```python
from build123d import *

# Parameters (mm, degrees)
F1_DEPTH = 3.048


with BuildPart() as f1:
    # F0 (on Front) → F1 (new body)
    with BuildSketch(Plane.XZ):
        with BuildLine():
            add(Edge.make_bspline(
                [(0, -29.2028061362), (0.1994290432, -29.2090684708), (0.3988582249, -29.2153378493), (0.5982729839, -29.2216137104)],
                knots=[0, 0, 0, 0, 0.0080246695, 0.0080246695, 0.0080246695, 0.0080246695], degree=3))
            Line((0, -29.2028061362), (0, -38.7278061362))
            Line((0, -38.7278061362), (9.525, -38.7278061362))
            ThreePointArc((9.525, -38.7278061362), (6.9434924632, -32.2075655415), (0.5982729839, -29.2216137104))
        make_face()
        with BuildLine():
            ThreePointArc((-9.525, -38.7278061362), (-6.7351920908, -31.9926140454), (0, -29.2028061362))
            Line((0, -29.2028061362), (0, -15.875))
            ThreePointArc((0, -15.875), (-11.0057082375, -11.4407172498), (-15.8630798211, -0.6150801499))
            add(Edge.make_bspline(
                [(-15.8630798211, -0.6150801499), (-15.5610688303, -14.0326352056), (-12.5430344151, -26.3802206709), (-9.525, -38.7278061362)],
                knots=[0.5347471817, 0.5347471817, 0.5347471817, 0.5347471817, 1, 1, 1, 1], degree=3))
        make_face()
        with BuildLine():
            Line((0, -38.7278061362), (0, -29.2028061362))
            ThreePointArc((0, -29.2028061362), (-6.7351920908, -31.9926140454), (-9.525, -38.7278061362))
            ThreePointArc((-9.525, -38.7278061362), (-6.7351920908, -45.4629982271), (0, -48.2528061362))
            add(Edge.make_bspline(
                [(0, -48.2528061362), (0.2131130588, -48.2456482665), (0.4262259719, -48.2384878681), (0.6393387432, -48.2313250094)],
                knots=[0, 0, 0, 0, 0.6396952306, 0.6396952306, 0.6396952306, 0.6396952306], degree=3))
            ThreePointArc((0.6393387432, -48.2313250094), (6.957561589, -45.2330318614), (9.525, -38.7278061362))
            Line((9.525, -38.7278061362), (0, -38.7278061362))
        make_face()
        with BuildLine():
            Line((0, -15.875), (0, -29.2028061362))
            ThreePointArc((0, -29.2028061362), (0.2992842663, -29.2075091909), (0.5982729839, -29.2216137104))
            add(Edge.make_bspline(
                [(0.5982729839, -29.2216137104), (4.3416181778, -29.339422014), (8.0798811955, -29.4595146085), (11.716745228, -29.5781777813)],
                knots=[0.0080246695, 0.0080246695, 0.0080246695, 0.0080246695, 0.1586610028, 0.1586610028, 0.1586610028, 0.1586610028], degree=3))
            add(Edge.make_bspline(
                [(15.8630798211, -0.6150801499), (15.6355353264, -10.7242843795), (13.866216965, -20.2261112434), (11.7167452282, -29.578177782)],
                knots=[0.5347471817, 0.5347471817, 0.5347471817, 0.5347471817, 0.8852831578, 0.8852831578, 0.8852831578, 0.8852831578], degree=3))
            ThreePointArc((15.8630798211, -0.6150801499), (11.0057082375, -11.4407172498), (0, -15.875))
        make_face()
        with BuildLine():
            ThreePointArc((0.5982729839, -29.2216137104), (0.2992842663, -29.2075091909), (0, -29.2028061362))
            add(Edge.make_bspline(
                [(0, -29.2028061362), (0.1994290432, -29.2090684708), (0.3988582249, -29.2153378493), (0.5982729839, -29.2216137104)],
                knots=[0, 0, 0, 0, 0.0080246695, 0.0080246695, 0.0080246695, 0.0080246695], degree=3))
        make_face()
        with BuildLine():
            ThreePointArc((-15.8630798211, -0.6150801499), (-11.0057082375, -11.4407172498), (0, -15.875))
            Line((0, -15.875), (0, 0))
            Line((0, 0), (0, 15.875))
            ThreePointArc((0, 15.875), (-11.2253201513, 11.2253201513), (-15.875, 0))
            add(Edge.make_bspline(
                [(-15.875, 0), (-15.8716656679, -0.2052784728), (-15.8676890566, -0.4103039216), (-15.8630798211, -0.6150801499)],
                knots=[0.5276465798, 0.5276465798, 0.5276465798, 0.5276465798, 0.5347471817, 0.5347471817, 0.5347471817, 0.5347471817], degree=3))
        make_face()
        with BuildLine():
            Line((0, 0), (0, -15.875))
            ThreePointArc((0, -15.875), (11.0057082375, -11.4407172498), (15.8630798211, -0.6150801499))
            add(Edge.make_bspline(
                [(15.875, 0), (15.8716656679, -0.2052784728), (15.8676890566, -0.4103039216), (15.8630798211, -0.6150801499)],
                knots=[0.5276465798, 0.5276465798, 0.5276465798, 0.5276465798, 0.5347471817, 0.5347471817, 0.5347471817, 0.5347471817], degree=3))
            ThreePointArc((15.875, 0), (11.2253201513, 11.2253201513), (0, 15.875))
            Line((0, 15.875), (0, 0))
        make_face()
        with BuildLine():
            add(Edge.make_bspline(
                [(0.5982729839, -29.2216137104), (4.3416181778, -29.339422014), (8.0798811955, -29.4595146085), (11.716745228, -29.5781777813)],
                knots=[0.0080246695, 0.0080246695, 0.0080246695, 0.0080246695, 0.1586610028, 0.1586610028, 0.1586610028, 0.1586610028], degree=3))
            ThreePointArc((0.5982729839, -29.2216137104), (6.9434924632, -32.2075655415), (9.525, -38.7278061362))
            add(Edge.make_bspline(
                [(11.7167452282, -29.578177782), (11.0133064179, -32.63874678), (10.2691532089, -35.6832764581), (9.525, -38.7278061362)],
                knots=[0.8852831578, 0.8852831578, 0.8852831578, 0.8852831578, 1, 1, 1, 1], degree=3))
        make_face()
        with BuildLine():
            add(Edge.make_bspline(
                [(11.7167452282, -29.578177782), (11.0133064179, -32.63874678), (10.2691532089, -35.6832764581), (9.525, -38.7278061362)],
                knots=[0.8852831578, 0.8852831578, 0.8852831578, 0.8852831578, 1, 1, 1, 1], degree=3))
            Line((9.525, -38.7278061362), (38.8504122414, -38.7278061362))
            ThreePointArc((38.8504122414, -38.7278061362), (41.0703889722, -33.2220061112), (46.4885436218, -30.7959535986))
            add(Edge.make_bspline(
                [(46.6014932618, -30.7924955428), (46.5682462049, -30.7929887265), (46.5283758233, -30.7939133608), (46.4885436218, -30.7959535986)],
                knots=[0.9751953485, 0.9751953485, 0.9751953485, 0.9751953485, 1, 1, 1, 1], degree=3))
            ThreePointArc((46.6014932618, -30.7924955428), (46.6427611197, -30.7916334188), (46.684032903, -30.7909859082))
            add(Edge.make_bspline(
                [(11.716745228, -29.5781777813), (30.5622726651, -30.1930674385), (46.6851234184, -30.7695755158), (46.684032903, -30.7909859082)],
                knots=[0.1586610028, 0.1586610028, 0.1586610028, 0.1586610028, 0.9392294066, 0.9392294066, 0.9392294066, 0.9392294066], degree=3))
        make_face()
        with BuildLine():
            Line((38.8504122414, -38.7278061362), (9.525, -38.7278061362))
            ThreePointArc((9.525, -38.7278061362), (6.957561589, -45.2330318614), (0.6393387432, -48.2313250094))
            add(Edge.make_bspline(
                [(0.6393387432, -48.2313250094), (16.0478252892, -47.7134357647), (31.455570606, -47.182685244), (46.8640654981, -46.6649408164)],
                knots=[0.6396952306, 0.6396952306, 0.6396952306, 0.6396952306, 46.8909606742, 46.8909606742, 46.8909606742, 46.8909606742], degree=3))
            ThreePointArc((46.8640654981, -46.6649408164), (41.2022412981, -44.3673261834), (38.8504122414, -38.7278061362))
        make_face()
        with BuildLine():
            ThreePointArc((-15.875, 0), (-15.8720196755, -0.3075978225), (-15.8630798211, -0.6150801499))
            add(Edge.make_bspline(
                [(-15.875, 0), (-15.8716656679, -0.2052784728), (-15.8676890566, -0.4103039216), (-15.8630798211, -0.6150801499)],
                knots=[0.5276465798, 0.5276465798, 0.5276465798, 0.5276465798, 0.5347471817, 0.5347471817, 0.5347471817, 0.5347471817], degree=3))
        make_face()
        with BuildLine():
            add(Edge.make_bspline(
                [(15.875, 0), (15.8716656679, -0.2052784728), (15.8676890566, -0.4103039216), (15.8630798211, -0.6150801499)],
                knots=[0.5276465798, 0.5276465798, 0.5276465798, 0.5276465798, 0.5347471817, 0.5347471817, 0.5347471817, 0.5347471817], degree=3))
            ThreePointArc((15.8630798211, -0.6150801499), (15.8720196755, -0.3075978225), (15.875, 0))
        make_face()
        with BuildLine():
            add(Edge.make_bspline(
                [(0, -48.2528061362), (0.2131130588, -48.2456482665), (0.4262259719, -48.2384878681), (0.6393387432, -48.2313250094)],
                knots=[0, 0, 0, 0, 0.6396952306, 0.6396952306, 0.6396952306, 0.6396952306], degree=3))
            ThreePointArc((0, -48.2528061362), (0.3198497567, -48.2474343398), (0.6393387432, -48.2313250094))
        make_face()
        with BuildLine():
            ThreePointArc((46.4885436218, -30.7959535986), (41.0703889722, -33.2220061112), (38.8504122414, -38.7278061362))
            ThreePointArc((38.8504122414, -38.7278061362), (41.2022412981, -44.3673261834), (46.8640654981, -46.6649408164))
            add(Edge.make_bspline(
                [(46.8640654981, -46.6649408164), (46.9909147503, -46.6606785252), (47.1177640532, -46.6564171153), (47.2446134078, -46.6521566014)],
                knots=[46.8909606742, 46.8909606742, 46.8909606742, 46.8909606742, 47.2717206688, 47.2717206688, 47.2717206688, 47.2717206688], degree=3))
            ThreePointArc((47.2446134078, -46.6521566014), (52.5597824651, -44.1766060381), (54.7254122414, -38.7278061362))
            ThreePointArc((54.7254122414, -38.7278061362), (52.3637244693, -33.078538551), (46.684032903, -30.7909859082))
            add(Edge.make_bspline(
                [(46.684032903, -30.7909859082), (46.6839826557, -30.7919724263), (46.6497004182, -30.7917804424), (46.6014932618, -30.7924955428)],
                knots=[0.9392294066, 0.9392294066, 0.9392294066, 0.9392294066, 0.9751953485, 0.9751953485, 0.9751953485, 0.9751953485], degree=3))
            ThreePointArc((46.6014932618, -30.7924955428), (46.5450122879, -30.7940235666), (46.4885436218, -30.7959535986))
        make_face()
        with BuildLine():
            ThreePointArc((-15.875, 0), (-11.2253201513, 11.2253201513), (0, 15.875))
            Line((0, 15.875), (0, 39.0321981638))
            ThreePointArc((0, 39.0321981638), (-6.7351920908, 41.822006073), (-9.525, 48.5571981638))
            add(Edge.make_bspline(
                [(-9.525, 48.5571981638), (-12.8238873086, 31.9057330322), (-16.1227746172, 15.2542679006), (-15.875, 0)],
                knots=[0, 0, 0, 0, 0.5276465798, 0.5276465798, 0.5276465798, 0.5276465798], degree=3))
        make_face()
        with BuildLine():
            Line((0, 39.0321981638), (0, 15.875))
            ThreePointArc((0, 15.875), (11.2253201513, 11.2253201513), (15.875, 0))
            add(Edge.make_bspline(
                [(9.525, 48.5571981638), (12.8238873086, 31.9057330322), (16.1227746172, 15.2542679006), (15.875, 0)],
                knots=[0, 0, 0, 0, 0.5276465798, 0.5276465798, 0.5276465798, 0.5276465798], degree=3))
            ThreePointArc((9.525, 48.5571981638), (6.7351920908, 41.822006073), (0, 39.0321981638))
        make_face()
        with BuildLine():
            add(Edge.make_bspline(
                [(46.684032903, -30.7909859082), (46.6839826557, -30.7919724263), (46.6497004182, -30.7917804424), (46.6014932618, -30.7924955428)],
                knots=[0.9392294066, 0.9392294066, 0.9392294066, 0.9392294066, 0.9751953485, 0.9751953485, 0.9751953485, 0.9751953485], degree=3))
            ThreePointArc((46.684032903, -30.7909859082), (46.6427611197, -30.7916334188), (46.6014932618, -30.7924955428))
        make_face()
        with BuildLine():
            add(Edge.make_bspline(
                [(46.6014932618, -30.7924955428), (46.5682462049, -30.7929887265), (46.5283758233, -30.7939133608), (46.4885436218, -30.7959535986)],
                knots=[0.9751953485, 0.9751953485, 0.9751953485, 0.9751953485, 1, 1, 1, 1], degree=3))
            ThreePointArc((46.4885436218, -30.7959535986), (46.5450122879, -30.7940235666), (46.6014932618, -30.7924955428))
        make_face()
        with BuildLine():
            add(Edge.make_bspline(
                [(46.8640654981, -46.6649408164), (46.9909147503, -46.6606785252), (47.1177640532, -46.6564171153), (47.2446134078, -46.6521566014)],
                knots=[46.8909606742, 46.8909606742, 46.8909606742, 46.8909606742, 47.2717206688, 47.2717206688, 47.2717206688, 47.2717206688], degree=3))
            ThreePointArc((46.8640654981, -46.6649408164), (47.0544161215, -46.6608309019), (47.2446134078, -46.6521566014))
        make_face()
        with BuildLine():
            ThreePointArc((-9.525, 48.5571981638), (-6.7351920908, 41.822006073), (0, 39.0321981638))
            ThreePointArc((0, 39.0321981638), (6.7351920908, 41.822006073), (9.525, 48.5571981638))
            ThreePointArc((9.525, 48.5571981638), (0, 58.0821981638), (-9.525, 48.5571981638))
        make_face()
    extrude(amount=F1_DEPTH)


solid = f1.part
```
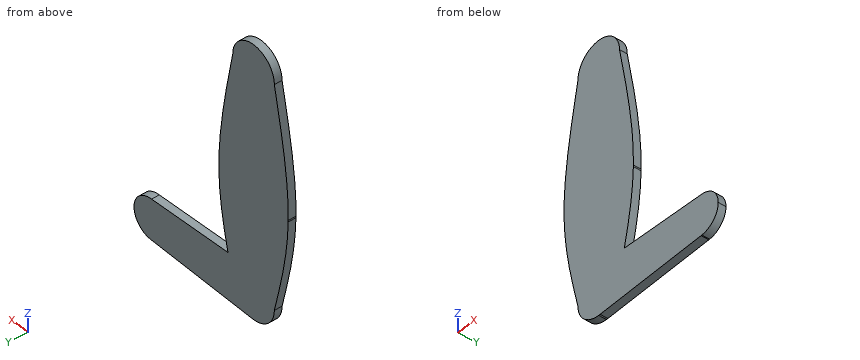
Source: CAD feature listing. Evaluate the final solid. Frame: model axes, mm. Give positions to 0.01 mm unless a question says otherwise; leave off trailing zeros. Loops run counter-clockwise (first coordinate to the right, second up) from the corner with the lowest first, then second, coordinate; pieces in that order, holes last. Notation, with made-up numbers: (65, 49) - (88, 49) arc R28 cw to (88, 67) - close; hole circle Ø8 at (53, 25). An arc over 180 degrees is marked (long way). Use CSV: the item, a comma, the result in double quotes.
1) Line query: line 1 (Z direction, x = 0.5, y = -0.15); line 2 (X direction, y = -1.7, z = 0.5); line 3 (X direction, y = -2.3, z = 33). Output: solid intervals per line, ascending.
Worked out:
line 1,"z = -48.24 to 58.07"
line 2,"x = -15.88 to 15.88"
line 3,"x = -12.51 to 12.51"
2) Pin query (flat end, axial travel): P1, Ø1.5, axis at x = 18, y = -2, coming from the -Z side; P2, Ø1, axis at y = -1, z = -0.5, coming from the -X side (3 decimals); P3, Ø1.5, axis at y = -1.5, z = 42.5, coming from the +X side. Return the tip coordinate at first contact, or that it passes through.
Worked out:
P1,"stops at z = -47.67"
P2,"stops at x = -15.875"
P3,"stops at x = 10.87"
3) Cut plane A-A (x = -4.5). Output: boundary loops of the cut face in (y, z).
Worked out:
outline,"(-3.05, -47.12) - (0, -47.12) - (0, 56.95) - (-3.05, 56.95) - close"
